Part model, mm, in its own coordinate system. A direction names the side the tool comes from. Give positions to 0.01 mm unless a question says otherwise; leave off trailing zeros. Order: outer loops, then holes, each group sorted by start corner. A loop starts at its lowest first (then second) coordinate and runs counter-clockwise, first axis right, second up. Notation, with made-up numbers: M 6.25,54 L 34.25,54 A15 ccw 34.25,67 Z; hole C 65.25,88 d2. An arc over 180 degrees is marked long. Answer as a JSON object with one key per item and string values.
from build123d import *

# Parameters (mm, degrees)
ESBO_O1_R                = 1.65
RESSALTO_EXTRUS_O1_DEPTH = 12
ESBO_O2_W                = 11
ESBO_O2_H                = 5
CORTE_EXTRUS_O1_DEPTH    = 25.355902775
FILETE1_R                = 5
ESBO_O3_R                = 1.65
CORTE_EXTRUS_O2_DEPTH    = 2.5
ESBO_O3_2_R              = 1.65
CORTE_EXTRUS_O3_DEPTH    = 27.184155514
RESSALTO_EXTRUS_O2_DEPTH = 3
FILETE2_R                = 5


with BuildPart() as part:
    # Esboço1 → Ressalto-extrusão1 (new body)
    with BuildSketch(Plane.XY):
        Polygon((0, 0), (-13.9, 0), (-13.9, -10), (-4, -16), (7, -16), (7, 0), (3, 0), (3, -10), (0, -10), align=None)
        with Locations((-9.9, -5)):
            Circle(ESBO_O1_R, mode=Mode.SUBTRACT)
    extrude(amount=RESSALTO_EXTRUS_O1_DEPTH)

    # Esboço2 → Corte-extrusão1 (cut, through all)
    with BuildSketch(Plane(origin=(0, 0, 0), x_dir=(1, 0, 0), z_dir=(0, 1, 0))):
        with Locations((-8.4, -6)):
            Rectangle(ESBO_O2_W, ESBO_O2_H)
    extrude(amount=-CORTE_EXTRUS_O1_DEPTH, mode=Mode.SUBTRACT)

    # Filete1
    filete1_edges = [part.edges().sort_by_distance(p)[0] for p in [
        (-4, -16, 1.75),
        (-13.9, -10, 10.25),
        (-13.9, -10, 1.75),
        (-13.9, 0, 1.75),
        (-13.9, 0, 10.25),
    ]]
    fillet(filete1_edges, radius=FILETE1_R)

    # Esboço3 → Corte-extrusão2 (cut)
    with BuildSketch(Plane.ZY.offset(-3)):
        Polygon((2.535898385, -5), (4.267949192, -8), (7.732050808, -8), (9.464101615, -5), (7.732050808, -2), (4.267949192, -2), align=None)
        with Locations(Location((6, -5, 0), (0, 0, 270))):
            Circle(ESBO_O3_R, mode=Mode.SUBTRACT)
    extrude(amount=-CORTE_EXTRUS_O2_DEPTH, mode=Mode.SUBTRACT)

    # Esboço3<2> → Corte-extrusão3 (cut, through all)
    with BuildSketch(Plane.ZY.offset(-3)):
        with Locations(Location((6, -5, 0), (0, 0, 270))):
            Circle(ESBO_O3_2_R)
    extrude(amount=-CORTE_EXTRUS_O3_DEPTH, mode=Mode.SUBTRACT)

    # Esboço4 → Ressalto-extrusão2 (add)
    with BuildSketch(Plane.XZ.offset(16)):
        with BuildLine():
            Line((7, 12), (-17.9, 12))
            Line((-17.9, 12), (-17.9, 0))
            Line((-17.9, 0), (-14.4, 0))
            Line((-14.4, 0), (-14.4, 4.5))
            ThreePointArc((-14.4, 4.5), (-15.9, 6), (-14.4, 7.5))
            Line((-14.4, 7.5), (-5.4, 7.5))
            ThreePointArc((-5.4, 7.5), (-3.9, 6), (-5.4, 4.5))
            Line((-5.4, 4.5), (-5.4, 0))
            Line((-5.4, 0), (7, 0))
            Line((7, 0), (7, 12))
        make_face()
    extrude(amount=-RESSALTO_EXTRUS_O2_DEPTH)

    # Filete2
    # the kernel refuses this fillet: 5 mm, written as the material it adds along each edge
    with BuildSketch(Plane(origin=(-8.95, -13, 12), x_dir=(-1, 0, 0), z_dir=(0, 0, -1))) as filete2_piece_1:
        with BuildLine():
            CenterArc((9.908595848, 4.907249128), FILETE2_R, 174.784336803, 84.162533203)
            Line((4.929297924, 5.361773258), (4.431368132, 5.407225671))
            ThreePointArc((4.431368132, 5.407225671), (2.282357722, 1.967907146), (-0.259150858, 0.427598916))
            Line((-0.259150858, 0.427598916), (0, -0.5))
            ThreePointArc((0, -0.5), (4.475, -0.5), (8.854140415, -0.490724913))
            Line((8.854140415, -0.490724913), (8.95, 0))
        make_face()
    extrude(amount=3.5)


solid = part.part
1. Cut at A-A on x = -5. Give the cut face in (y, z), plus the area to 3 significant figures.
Worked answers:
{"outline": "M -16,0 L 0,0 L 0,3.5 L -13,3.5 L -13,4.55 L -16,4.55 Z; M -16,7.45 L -13,7.45 L -13,8.5 L 0,8.5 L 0,12 L -16,12 Z", "area": "118 mm^2"}
2. Which spindle directions (+Z, -Z, +X, -X, +Y, -Y) get a long thin tool onto all of the face, cutting with end or side? Do faces 5 (the flat face through (-2.9, -6, 6)), 6 (the flat face through (-10, -15, 7.5)), 7 (the flat face through (4.2, -3.5, 8.6)), 8 (the flat face through (-13.9, -6, 10)), 9 (the flat face through (3, -1.6, 5.9)). Say none if no direction does.
Worked answers:
{"face 5": "-X, +Y", "face 6": "+Y, -Y", "face 7": "none", "face 8": "+Z, -Z, -X, +Y", "face 9": "+Z, -Z, +Y"}
3. Pin check, flat tips, straight feed: P1, Ø1.8, axis at y = -5, z = 7, coming from the -X side; P2, Ø4, axis at x = -13, z = 5, coming from the +Y side; P3, Ø2.5, axis at y = -6.5, z = 1, coming from the -X side. Stop position of each tip, or through.
Worked answers:
{"P1": "stops at x = -2.9", "P2": "stops at y = -0.84", "P3": "stops at x = -13.9"}
4. Two-plate mould, pull along Y, no slides. Class faces 1 (the flat face through (-7, -7, 3.5)), 2 (the flat face through (4.2, -3.5, 3.4)), 3 (the flat face through (-8.49, -13.28, 1.73)), 4 (the cylindrical face through (-10.3, -6.6, 1.7)): +Y half, -Y half, draft (parallel to the pull), parting line (faces both ways), or undercut.
Worked answers:
{"face 1": "draft", "face 2": "undercut", "face 3": "-Y half", "face 4": "undercut"}
5. Cut at C-C on z = 10.5. Give the cut face in (x, y), plus the area to 3 significant figures.
Worked answers:
{"outline": "M -17.9,-16 L 7,-16 L 7,0 L 3,0 L 3,-10 L 0,-10 L 0,0 L -8.9,0 A5 ccw -13.9,-5 L -13.9,-7.18 A5 ccw -13.88,-7.64 A5 cw -17.9,-13 Z; hole C -9.9,-5 d3.3", "area": "307 mm^2"}
6. Cut at B-B on y = -1.5. Give the cut face in (x, z), plus the area to 3 significant figures.
Worked answers:
{"outline": "M -12.47,0 L 0,0 L 0,12 L -12.47,12 L -12.47,8.5 L -2.9,8.5 L -2.9,3.5 L -12.47,3.5 Z; M 3,0 L 7,0 L 7,12 L 3,12 Z", "area": "150 mm^2"}
7. Cut at D-D on x = -10.5. Give the cut face in (y, z), plus the area to 3 significant figures.
Worked answers:
{"outline": "M -16,7.5 L -13,7.5 L -13,8.5 L -6.54,8.5 L -6.54,12 L -16,12 Z; M -12.06,0 L -6.54,0 L -6.54,3.5 L -12.06,3.5 Z; M -3.46,0 L -0.26,0 L -0.26,3.5 L -3.46,3.5 Z; M -3.46,8.5 L -0.26,8.5 L -0.26,12 L -3.46,12 Z", "area": "77.9 mm^2"}
8. Probe line 1 along Z through (x, y) = (6.6, -5); line 2 along Y through (x, z) = (4, 6.75); line 3 along Z through (x, y) = (-3.5, -2.5). List the from-to ranges inside material, lowest first.
Worked answers:
{"line 1": "z = 0 to 4.35, 7.65 to 12", "line 2": "y = -16 to -8, -2 to 0", "line 3": "z = 0 to 3.5, 8.5 to 12"}
